Part model, mm, in its own coordinate system. A direction names the side the tool comes from. Round coordinates to 2 decimals unless told otherwise and drop trailing zeros. Order: outer loops, then holes, each group sorted by start corner. A loop starts at its lowest first (then second) coordinate and runs counter-clockwise, first axis right, second up. Notation, with made-up numbers: (63, 26) - (112, 26) arc R29 cw to (112, 61) - close; hole circle Ø11 at (58, 66). An arc over 180 degrees is marked (long way). Return JSON: item names as keys, results as strings. Group by question number.
Item 1: Saw through at B-B on z = 0. List the corners of the cut face in (x, y).
Item 2: Drop flat-ended pins along their axis: pin 1 (20 mm diameter, centred on x = -17.68, z = 0, fed in from +Y); pin 2 (6 mm diameter, centred on x = -21, y = 46.5, fed in from +Z); pin 3 (2 mm diameter, centred on x = -28.5, z = 18.5, fed in from -Y). Give the stop position or say it passes through.
Item 3: Probe probe 1 along Y at (x, z) = (-19.5, 0); probe 2 along Z at (x, y) = (-13.5, -56.5); probe 3 along Y at (x, z) = (5.5, 16). List the from-to ranges inside material, lowest first.
Item 4: Saw through at C-C on x = -8. List the corners of the cut face in (y, z).
Item 5: Two-plate mould, pull along X, no slides. Class faces 1 (the face through (-10.983, 64.639, -14.354)), 2 (the face through (-37.683, 20.4, -64)), 3 (the face through (-29.606, 90.14, -3.755)): released by +X, released by -X, zero draft, split by the parting line, or undercut.
Item 6: Tool access for faces 4 (the face through (-18, 80, 0)), 5 (the face through (-29.606, -89.811, -3.755)), 6 (the face through (-7.29, -30.04, 95.38)): list every direction of +Z, -Z, +X, -X, +Y, -Y with a clear straight run to the whole face (end or side of a thin tool).
Item 7: Saw through at A-A on y = 0. List the corners of the cut face in (x, z).
Item 8: Saw through at D-D on x = -25.5. List the corners of the cut face in (y, z).
```python
from build123d import *

# Parameters (mm, degrees)
CHAMFER_1_SIZE = 2
SKETCH_2_W     = 12.5
SKETCH_2_H     = 20


with BuildPart() as part:
    # Эскиз1 → Повернуть1 (revolve)
    with BuildSketch(Plane.XY, mode=Mode.PRIVATE) as revolve_1_sk:
        Polygon((-37.682926829, -65), (-37.682926829, -100), (22.317073171, -100), (22.317073171, -90), (-12.682926829, -65), align=None)
    revolve(revolve_1_sk.sketch.rotate(Axis((-193.536585366, 0, 0), (1, 0, 0)), 270), axis=Axis((-193.536585366, 0, 0), (1, 0, 0)))

    # Фаска1
    chamfer_1_edges = [part.edges().sort_by_distance(p)[0] for p in [
        (22.317073171, 0, -100),
        (-37.682926829, 0, -100),
        (-37.682926829, 0, -65),
    ]]
    chamfer(chamfer_1_edges, length=CHAMFER_1_SIZE)

    # Эскиз2 → Вырез-Повернуть1 (revolve, cut)
    with BuildSketch(Plane.XY, mode=Mode.PRIVATE) as cut_revolve_1_sk:
        Polygon((-5.182926829, -99.902279859), (-5.182926829, -79.902279859), (-17.682926829, -79.902279859), (-17.682926829, -99.902279859), (-17.682926829, -106.132104806), (-5.182926829, -106.132104806), align=None)
        with Locations((-11.432926829, 90)):
            Rectangle(SKETCH_2_W, SKETCH_2_H)
    revolve(cut_revolve_1_sk.sketch.rotate(Axis((-17.682926829, 126.68088459, 0), (0, -1, 0)), 180), axis=Axis((-17.682926829, 126.68088459, 0), (0, -1, 0)), mode=Mode.SUBTRACT)


solid = part.part
```
Filled in:
{
 "1": {"outline": "(-37.68, -98) - (-35.68, -100) - (-30.18, -100) - (-30.18, -79.9) - (-5.18, -79.9) - (-5.18, -100) - (20.32, -100) - (22.32, -98) - (22.32, -90) - (-12.68, -65) - (-35.68, -65) - (-37.68, -67) - close; (-37.68, 67) - (-35.68, 65) - (-12.68, 65) - (22.32, 90) - (22.32, 98) - (20.32, 100) - (-5.18, 100) - (-5.18, 80) - (-30.18, 80) - (-30.18, 100) - (-35.68, 100) - (-37.68, 98) - close"},
 "2": {"pin 1": "stops at y = 80", "pin 2": "stops at z = 90.04", "pin 3": "stops at y = -98.46"},
 "3": {"probe 1": "y = -79.9 to -65, 65 to 80", "probe 2": "z = -82.51 to -32.14, 32.14 to 82.51", "probe 3": "y = -98.71 to -76.33, 76.33 to 98.71"},
 "4": {"outline": "(-99.69, -7.91) arc R100 ccw to (99.69, -7.91) - (80, -7.91) - (80, 7.91) - (99.69, 7.91) arc R100 ccw to (-99.69, 7.91) - (-79.9, 7.91) - (-79.9, -7.91) - close; hole circle Ø136.69 at (0, 0)"},
 "5": {"face 1": "released by +X", "face 2": "released by -X", "face 3": "undercut"},
 "6": {"face 4": "+Y", "face 5": "-Y", "face 6": "+X, -X"},
 "7": {"outline": "(-37.68, -98) - (-35.68, -100) - (20.32, -100) - (22.32, -98) - (22.32, -90) - (-12.68, -65) - (-35.68, -65) - (-37.68, -67) - close; (-37.68, 67) - (-35.68, 65) - (-12.68, 65) - (22.32, 90) - (22.32, 98) - (20.32, 100) - (-35.68, 100) - (-37.68, 98) - close"},
 "8": {"outline": "(-99.52, -9.75) arc R100 ccw to (99.52, -9.75) - (80, -9.75) - (80, 9.75) - (99.52, 9.75) arc R100 ccw to (-99.52, 9.75) - (-79.9, 9.75) - (-79.9, -9.75) - close; hole circle Ø130 at (0, 0)"}
}
